Autodesk Inventor part; units mm, degrees
ref_plane "Arbeitsebene1" through (0, 28, 0) normal (0, 1, 0) x (-1, 0, 0)
ref_plane "YZ Plane" through (0, 0, 0) normal (1, 0, 0) x (0, 1, 0)
ref_plane "XY Plane" through (0, 0, 0) normal (0, 0, 1) x (1, 0, 0)
sketch "Skizze1" plane through (0, 0, 0) normal (0, 1, 0) x (-1, 0, 0)
  line L0 (0, 0) -> (28, 0)
  line L1 (28, 0) -> (28, -38)
  line L2 (28, -38) -> (58, -38)
  line L3 (58, -38) -> (58, -60)
  line L4 (58, -60) -> (0, -60)
  line L5 (0, -60) -> (0, 0)
  dimension "d0" = 116
  dimension "d1" = 56
  dimension "d2" = 22
  dimension "d3" = 38
revolve "Umdrehung1" add sketch "Skizze1" angle 360 about axis through (0, 0, -60) along (0, 0, 1)
sketch "Skizze2" plane through (0, 0, 0) normal (0, 0, 1) x (1, 0, 0)
  circle A0 centre (0, 0) radius 14
  dimension "d5" = 28
extrude "Extrusion1" cut sketch "Skizze2" against normal up to surface (60 mm away)
ref_plane "Arbeitsebene1" through (0, 28, 0) normal (0, 1, 0) x (-1, 0, 0)
sketch "Skizze3" plane through (0, 28, 0) normal (0, 1, 0) x (-1, 0, 0)
  point P0 (0, 0)
  point P1 (0, -12)
  dimension "d9" = 12
hole "Bohrung1" at (0, 28, -12) direction (0, -1, 0) diameter 10 end through all
sketch "Skizze4" plane through (0, 0, -60) normal (0, 0, -1) x (-1, 0, 0)
  circle A0 centre (0, 0) radius 44 construction
  circle A1 centre (0, 0) radius 14
  line L0 (0, 0) -> (0, 62.7079) construction
  line L1 (0, 0) -> (-33.1711, 57.4541) construction
  line L2 (0, 0) -> (35.197, 60.963) construction
  point P0 (-22, 38.1051)
  point P1 (22, 38.1051)
  dimension "d17" = 88
  dimension "d18" = 30
  dimension "d19" = 30
hole "Bohrung2" at (22, 38.1051, -60) at (-22, 38.1051, -60) direction (0, 0, 1) diameter 10.106 depth 22
pattern_circular "Runde Anordnung1" count 6 over 360 about axis through (0, 0, -49) along (0, 0, 1) of "Bohrung2"
properties part number "cover"
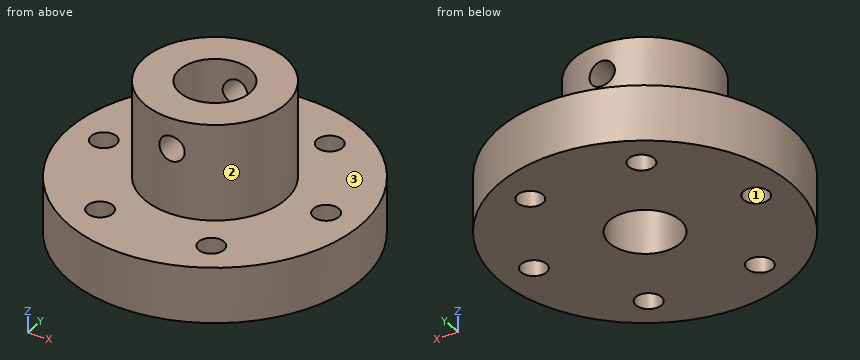
Work out the finished part from the listing and answer in its coordinate system (mm). Face numbers are marked on the shaded views. Round coordinates to 2 decimals unless told otherwise and drop trailing zeros. Write each loop counter-clockwise with the first axis right and the second up, starting at its lowest first coordinate (ties: lowest second). Pieces come first, ordered by that corner, then holes.
1) Determine the mould class of the marked faces 1, 2 and 3 for opening direction X: pulls with the +X half, pulls with the -X half, needs draft (parallel to the pull), parting line crosses it, or undercut.
2) A cutting plane is placed at B-B on y = 0. Determine the outline of the cut face in (x, z), and give its area (3 significant figures).
3) A cutting plane is placed at A-A on x = -22. Determine the outline of the cut face in (y, z), and give its area (3 significant figures).
4) A cutting plane is placed at D-D on y = 18.5. Determine the outline of the cut face in (x, z).
5) Flat-ended cylindrical pins translate along their axes: P1, Ø16, axis at x = 0, z = -12, coming from the +Y side; P2, Ø1.5, axis at y = 15.5, z = -28.5, coming from the -X side; P3, Ø5, axis at y = 16, z = -31.5, coming from the -X side; P4, Ø8, axis at x = 44, y = 0, coming from the +Z side. Find the tip coordinate at first contact, or state that the pin passes through.
6) Consider probe 1 along Z at (x, y) = (0, 21.5); probe 2 along Z at (x, y) = (-39, 29); probe 3 along X at (y, z) = (-19, -12). Determine where each line is inside the solid, lowest interval first.
7) A cutting plane is placed at C-C on x = -7. Determine the outline of the cut face in (y, z).
Entries:
1. face 1: undercut
1. face 2: parting line crosses it
1. face 3: needs draft
2. outline: (-58, -60) - (-49.05, -60) - (-49.05, -38) - (-58, -38) - close; (-38.95, -60) - (-14, -60) - (-14, 0) - (-28, 0) - (-28, -38) - (-38.95, -38) - close; (14, -60) - (38.95, -60) - (38.95, -38) - (28, -38) - (28, 0) - (14, 0) - close; (49.05, -60) - (58, -60) - (58, -38) - (49.05, -38) - close
2. area: 2,560 mm2
3. outline: (-53.67, -60) - (-43.16, -60) - (-43.16, -38) - (-53.67, -38) - close; (-33.05, -60) - (33.05, -60) - (33.05, -38) - (17.32, -38) - (17.32, 0) - (-17.32, 0) - (-17.32, -38) - (-33.05, -38) - close; (43.16, -60) - (53.67, -60) - (53.67, -38) - (43.16, -38) - close
3. area: 3,230 mm2
4. outline: (-54.97, -60) - (54.97, -60) - (54.97, -38) - (21.02, -38) - (21.02, 0) - (-21.02, 0) - (-21.02, -38) - (-54.97, -38) - close; hole circle Ø10 at (0, -12)
5. P1: stops at y = 28
5. P2: stops at x = -23.8
5. P3: stops at x = -24.53
5. P4: passes through
6. probe 1: z = -60 to -17, -7 to 0
6. probe 2: z = -60 to -38
6. probe 3: x = -20.57 to -5, 5 to 20.57
7. outline: (-57.58, -60) - (-12.12, -60) - (-12.12, 0) - (-27.11, 0) - (-27.11, -38) - (-57.58, -38) - close; (12.12, -60) - (57.58, -60) - (57.58, -38) - (27.11, -38) - (27.11, 0) - (12.12, 0) - close
